```python
from build123d import *

# Parameters (mm, degrees)
EXTRUDE_THIN1_DEPTH  = 15
SKETCH2_R            = 6.1
CUT_EXTRUDE1_DEPTH   = 62.306626885
FILLET1_R            = 12
FILLET1_OF_MIRROR1_R = 12


with BuildPart() as part:
    # Sketch1 → Extrude-Thin1 (new, symmetric)
    with BuildSketch(Plane.XY):
        Polygon((-55, 4.5), (-28, 4.5), (-28, 9.5), (-25.5, 9.5), (-25.5, 16), (-22, 16), (-22, 21.5), (-16.5, 21.5), (-16.5, 27.05), (0, 27.05), (0, 30.05), (-19.5, 30.05), (-19.5, 24.5), (-25, 24.5), (-25, 19), (-28.5, 19), (-28.5, 12.5), (-31, 12.5), (-31, 7.5), (-55, 7.5), align=None)
    extrude_thin1 = extrude(amount=EXTRUDE_THIN1_DEPTH, both=True)

    # Sketch2 → Cut-Extrude1 (cut, through all)
    with BuildSketch(Plane(origin=(0, 7.5, 0), x_dir=(1, 0, 0), z_dir=(0, 1, 0))):
        with Locations(Location((-44, 0, 0), (0, 0, 270))):
            Circle(SKETCH2_R)
    cut_extrude1 = extrude(amount=-CUT_EXTRUDE1_DEPTH, mode=Mode.SUBTRACT)

    # Fillet1
    fillet1_edges = [part.edges().sort_by_distance(p)[0] for p in [
        (-55, 6, -15),
        (-55, 6, 15),
    ]]
    fillet(fillet1_edges, radius=FILLET1_R)

    # Mirror1: Extrude-Thin1, Cut-Extrude1 across plane
    add(extrude_thin1.mirror(Plane(origin=(0, 30.05, 15), x_dir=(0, 0, 1), z_dir=(1, 0, 0))))
    add(cut_extrude1.mirror(Plane(origin=(0, 30.05, 15), x_dir=(0, 0, 1), z_dir=(1, 0, 0))), mode=Mode.SUBTRACT)

    # Fillet1 of Mirror1
    fillet1_of_mirror1_edges = [part.edges().sort_by_distance(p)[0] for p in [
        (55, 6, -15),
        (55, 6, 15),
    ]]
    fillet(fillet1_of_mirror1_edges, radius=FILLET1_OF_MIRROR1_R)


solid = part.part
```
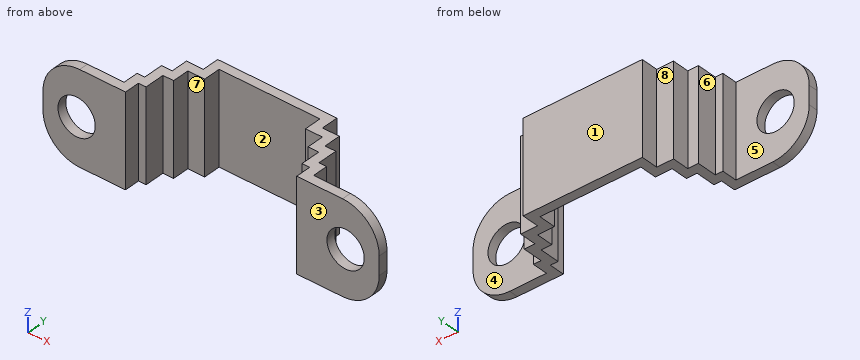
Verification items for the finished model (mm, model axes). Face numbers are marked on the shaded views. A direction names the side the tool comes from. Coordinates: 2 decimals unless noted, no trailing zeros. Loops run counter-clockwise (first coordinate to the right, second up) from the corner with the lowest first, then second, coordinate; pieces in that order, holes last. Notation, with made-up numbers: (57.25, 59) - (93.25, 59) arc R22 ccw to (93.25, 83) - close; hole circle Ø10 at (-4, 63.5). An arc over 180 degrees is marked (long way). Return JSON: item names as keys, results as strings.
1. Thickness scan on L1, parallel to X at y = 5.85, z = 0; L2, parallel to X at y = 9, z = -13; L3, parallel to X at y = 19.75, z = 9. Record the ranges inside material, lowest first.
Established:
{"L1": "x = -55 to -50.1, -37.9 to -28, 28 to 37.9, 50.1 to 55", "L2": "x = -31 to -28, 28 to 31", "L3": "x = -25 to -22, 22 to 25"}
2. Go/stop test with flat-tipped pins: pin 1 (4.5 mm diameter, centred on y = 19, z = 1, fed in from +X); pin 2 (0.8 mm diameter, centred on x = 29.5, z = -5, fed in from +Y); pin 3 (1 mm diameter, centred on y = 25.5, z = 0, fed in from +X); pin 4 (5 mm diameter, centred on x = 24, y = 13.5, fed in from +Z). Record where each tip stops, or that it passes through.
Established:
{"pin 1": "stops at x = 28.5", "pin 2": "stops at y = 12.5", "pin 3": "stops at x = 19.5", "pin 4": "stops at z = 15"}
3. Section check C-C, the plane z = 0. Count the separate pieces of the cut face and the enclosed holes in it, then the cut area to 3 significant figures.
Established:
{"separate pieces": "3", "enclosed holes": "0", "area": "392 mm2"}
4. Tool access check on the marked faces 1, 2, 3, 4 and 5. Record the directions out of +Z, -Z, +X, -X, +Y, -Y that give a thin tool (end or side, any length) a straight path to the whole face; none if there is none.
Established:
{"face 1": "+Z, -Z, +X, -X, +Y", "face 2": "+Z, -Z, -Y", "face 3": "+Z, -Z, +X, -X, -Y", "face 4": "+Z, -Z, +X, +Y", "face 5": "+Z, -Z, -X, +Y"}
5. Section check D-D, the plane x = -12. Record the boundary of the cut face in (y, z).
Established:
{"outline": "(27.05, -15) - (30.05, -15) - (30.05, 15) - (27.05, 15) - close"}
6. Mould release check, pull along X, two halves, no side actions. Record for the marked faces 6, 7 and 8: +X half, -X half, draft (parallel to the pull), parting line (faces both ways), or undercut.
Established:
{"face 6": "-X half", "face 7": "undercut", "face 8": "draft"}
7. Section check A-A, the plane y = 11. Record the boundary of the cut face in (x, z).
Established:
{"outline": "(-31, -15) - (-25.5, -15) - (-25.5, 15) - (-31, 15) - close; (25.5, -15) - (31, -15) - (31, 15) - (25.5, 15) - close"}
8. Section check B-B, the plane x = -44. Record the boundary of the cut face in (y, z).
Established:
{"outline": "(4.5, -14.96) - (7.5, -14.96) - (7.5, -6.1) - (4.5, -6.1) - close; (4.5, 6.1) - (7.5, 6.1) - (7.5, 14.96) - (4.5, 14.96) - close"}
